Source: CAD feature listing. Evaluate the final solid. Frame: model axes, mm. Face numbers are marked on the shaded views. Round coordinates to 2 decimals unless told otherwise and drop trailing zeros. Loops run counter-clockwise (first coordinate to the right, second up) from the corner with the lowest first, then second, coordinate; pieces in that order, holes last. Notation, with made-up numbers: M 29,-19.5 L 60,-19.5 A11 ccw 60,-6.5 Z; hole C 4.5,54.5 d8. An arc over 180 degrees is marked long. One line per item, written item: value.
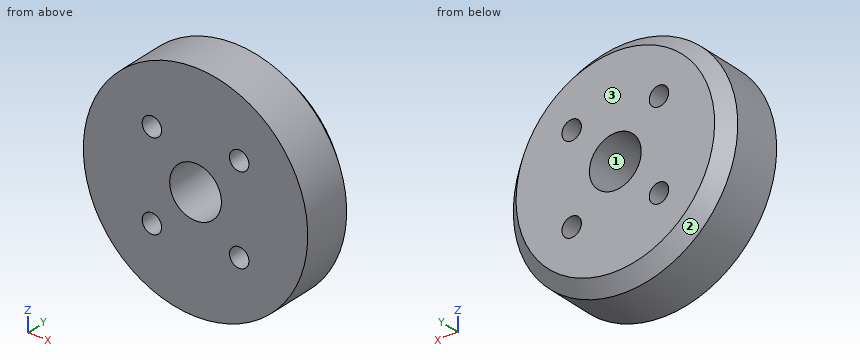
from build123d import *

# Parameters (mm, degrees)
SKETCH_1_R          = 17.35
EXTRUDE_1_DEPTH     = 9.6
CHAMFER_1_SIZE      = 2
SKETCH_2_R          = 4
SKETCH_2_R_2        = 1.5
CUT_EXTRUDE_1_DEPTH = 9.6


with BuildPart() as part:
    # 草图1 → 凸台-拉伸1 (new body)
    with BuildSketch(Plane(origin=(0, 0, 0), x_dir=(1, 0, 0), z_dir=(0, 1, 0))):
        with Locations(Location((0, 0, 0), (0, 0, 270))):
            Circle(SKETCH_1_R)
    extrude(amount=EXTRUDE_1_DEPTH)

    # 倒角1
    chamfer_1_edges = [part.edges().sort_by_distance(p)[0] for p in [
        (0, 9.6, -17.35),
    ]]
    chamfer(chamfer_1_edges, length=CHAMFER_1_SIZE)

    # 草图2 → 切除-拉伸1 (cut)
    with BuildSketch(Plane(origin=(0, 9.6, 0), x_dir=(1, 0, 0), z_dir=(0, 1, 0))):
        with Locations(Location((0, 0, 0), (0, 0, 270))):
            Circle(SKETCH_2_R)
        with Locations(Location((-6.75, 6.75, 0), (0, 0, 270))):
            Circle(SKETCH_2_R_2)
        with Locations(Location((6.75, 6.75, 0), (0, 0, 270))):
            Circle(SKETCH_2_R_2)
        with Locations(Location((6.75, -6.75, 0), (0, 0, 270))):
            Circle(SKETCH_2_R_2)
        with Locations(Location((-6.75, -6.75, 0), (0, 0, 270))):
            Circle(SKETCH_2_R_2)
    extrude(amount=-CUT_EXTRUDE_1_DEPTH, mode=Mode.SUBTRACT)


solid = part.part
1. Section query C-C (y = 2.75). Return the cut outline in (x, z), and give its area (3 significant figures).
Report:
outline: C 0,0 d34.7; hole C -6.75,-6.75 d3; hole C -6.75,6.75 d3; hole C 0,0 d8; hole C 6.75,-6.75 d3; hole C 6.75,6.75 d3
area: 867 mm2
2. Section query A-A (z = 0). Return the cut outline in (x, y).
Report:
outline: M -17.35,0 L -4,0 L -4,9.6 L -15.35,9.6 L -17.35,7.6 Z; M 4,0 L 17.35,0 L 17.35,7.6 L 15.35,9.6 L 4,9.6 Z
3. Pull-direction query (X, two-part tool) for the marked faces 1, 2 and 3; classes: released by +X, released by -X, zero draft, split by the parting line, or undercut.
Report:
face 1: undercut
face 2: split by the parting line
face 3: zero draft
4. Pin query (flat end, axial travel): pin 1 (1 mm diameter, centred on y = 5.5, z = 6.5, fed in from -X); pin 2 (1.8 mm diameter, centred on x = 6.75, z = 6.75, fed in from +Y); pin 3 (3 mm diameter, centred on y = 3.5, z = 11.5, fed in from +X); pin 4 (1.5 mm diameter, centred on x = -11, y = 8, fed in from +Z). Return the tip coordinate at first contact, or that it passes through.
Report:
pin 1: stops at x = -16.28
pin 2: passes through
pin 3: stops at x = 14.18
pin 4: stops at z = 13.91
5. Ray query, line 1 (X direction, y = 5.75, z = 6.75); line 2 (Z direction, x = 8, y = 7.5); line 3 (X direction, y = 6.75, z = 3.5). Return the intervals inside material, ascending. Write a range as [from, to].
Report:
line 1: x = [-15.98, -8.25], [-5.25, 5.25], [8.25, 15.98]
line 2: z = [-15.4, -7.58], [-5.92, 5.92], [7.58, 15.4]
line 3: x = [-16.99, -1.94], [1.94, 16.99]
6. Section query D-D (y = 8.75). Return the cut outline in (x, z).
Report:
outline: C 0,0 d32.4; hole C -6.75,-6.75 d3; hole C -6.75,6.75 d3; hole C 0,0 d8; hole C 6.75,-6.75 d3; hole C 6.75,6.75 d3
7. Section query B-B (x = 0). Return the cut outline in (y, z).
Report:
outline: M 0,-17.35 L 7.6,-17.35 L 9.6,-15.35 L 9.6,-4 L 0,-4 Z; M 0,4 L 9.6,4 L 9.6,15.35 L 7.6,17.35 L 0,17.35 Z
